Autodesk Inventor part; units mm, degrees
ref_plane "dia1_XY" through (-3.175, 3.9624, 0) normal (1, 0, 0) x (0, 0, -1)
ref_plane "dia1_YZ" through (-3.175, 3.9624, 0) normal (0, 0, -1) x (0, 1, 0)
ref_plane "dia1_ZX" through (-3.175, 3.9624, 0) normal (0, 1, 0) x (1, 0, 0)
sketch "Sketch_1" plane through (0, 0, 0) normal (0, 0, 1) x (1, 0, 0)
  line L0 (114.1984, 0) -> (-3.175, 0)
  line L1 (-3.175, 0) -> (-3.175, 3.9624)
  line L2 (-3.175, 3.9624) -> (92.075, 3.9624)
  line L3 (92.075, 3.9624) -> (92.075, 13.5572)
  line L4 (92.075, 13.5572) -> (114.1984, 13.5572)
  line L5 (114.1984, 13.5572) -> (114.1984, 0)
  line L6 (114.1984, 0) -> (-3.175, 0)
revolve "Revolution1" add sketch "Sketch_1" angle 360 about axis through (114.1984, 0, 0) along (1, 0, 0)
sketch "Sketch_3" plane through (0, 0, 0) normal (0, 0, 1) x (1, 0, 0)
  line L0 (-3.175, 0) -> (-15.875, 0)
  line L1 (-15.875, 0) -> (-15.875, 3.3388)
  line L2 (-15.875, 3.3388) -> (-15.2451, 3.9688)
  line L3 (-15.2451, 3.9688) -> (-3.175, 3.9688)
  line L4 (-3.175, 3.9688) -> (-3.175, 0)
  line L5 (-3.175, 0) -> (-15.875, 0)
revolve "Revolution2" add sketch "Sketch_3" angle 360 about axis through (-3.175, 0, 0) along (1, 0, 0)
thread "Thread1"
sketch "Sketch_10" plane through (-3.175, 0, 0) normal (1, 0, 0) x (0, 0, -1)
  line L0 (-7.9248, -7.9248) -> (7.9248, -7.9248)
  line L1 (7.9248, -7.9248) -> (7.9248, 7.9248)
  line L2 (7.9248, 7.9248) -> (-7.9248, 7.9248)
  line L3 (-7.9248, 7.9248) -> (-7.9248, -7.9248)
  line L4 (-3.175, -3.9624) -> (3.175, -3.9624)
  line L5 (3.175, -3.9624) -> (3.175, 3.9624)
  line L6 (3.175, 3.9624) -> (-3.175, 3.9624)
  line L7 (-3.175, 3.9624) -> (-3.175, -3.9624)
extrude "Extrusion1" cut sketch "Sketch_10" along normal blind 3.175
ref_plane "dia1_XY" through (-3.175, 3.9624, 0) normal (1, 0, 0) x (0, 0, -1)
ref_plane "dia1_YZ" through (-3.175, 3.9624, 0) normal (0, 0, -1) x (0, 1, 0)
ref_plane "dia1_ZX" through (-3.175, 3.9624, 0) normal (0, 1, 0) x (1, 0, 0)
ref_plane "dia12_XY" through (0, 0, 14.1351) normal (1, 0, 0) x (0, 0, -1)
ref_plane "dia12_YZ" through (0, 0, 14.1351) normal (0, 0, -1) x (0, 1, 0)
ref_plane "dia12_ZX" through (0, 0, 14.1351) normal (0, 1, 0) x (1, 0, 0)
ref_plane "dia2_XY" through (-3.175, -3.9624, 0) normal (1, 0, 0) x (0, 0, -1)
ref_plane "dia2_YZ" through (-3.175, -3.9624, 0) normal (0, 0, -1) x (0, 1, 0)
ref_plane "dia2_ZX" through (-3.175, -3.9624, 0) normal (0, 1, 0) x (1, 0, 0)
ref_plane "dia22_XY" through (0, 0, -14.1351) normal (1, 0, 0) x (0, 0, -1)
ref_plane "dia22_YZ" through (0, 0, -14.1351) normal (0, 0, -1) x (0, 1, 0)
ref_plane "dia22_ZX" through (0, 0, -14.1351) normal (0, 1, 0) x (1, 0, 0)
ref_plane "rl1_XY" through (-15.875, 0, 0) normal (1, 0, 0) x (0, 0, -1)
ref_plane "rl1_YZ" through (-15.875, 0, 0) normal (0, 0, -1) x (0, 1, 0)
ref_plane "rl1_ZX" through (-15.875, 0, 0) normal (0, 1, 0) x (1, 0, 0)
ref_plane "rl2_XY" through (-3.175, 0, 0) normal (1, 0, 0) x (0, 0, -1)
ref_plane "rl2_YZ" through (-3.175, 0, 0) normal (0, 0, -1) x (0, 1, 0)
ref_plane "rl2_ZX" through (-3.175, 0, 0) normal (0, 1, 0) x (1, 0, 0)
ref_plane "rod_cp_XY" through (0, 0, 0) normal (1, 0, 0) x (0, 0, -1)
ref_plane "rod_cp_YZ" through (0, 0, 0) normal (0, 0, -1) x (0, 1, 0)
ref_plane "rod_cp_ZX" through (0, 0, 0) normal (0, 1, 0) x (1, 0, 0)
ref_plane "thd1_XY" through (-15.875, 3.9688, 0) normal (1, 0, 0) x (0, 0, -1)
ref_plane "thd1_YZ" through (-15.875, 3.9688, 0) normal (0, 0, -1) x (0, 1, 0)
ref_plane "thd1_ZX" through (-15.875, 3.9688, 0) normal (0, 1, 0) x (1, 0, 0)
ref_plane "thd2_XY" through (-15.875, -3.9688, 0) normal (1, 0, 0) x (0, 0, -1)
ref_plane "thd2_YZ" through (-15.875, -3.9688, 0) normal (0, 0, -1) x (0, 1, 0)
ref_plane "thd2_ZX" through (-15.875, -3.9688, 0) normal (0, 1, 0) x (1, 0, 0)
ref_plane "to_rod_clevis_XY" through (-20.701, 0, 0) normal (1, 0, 0) x (0, 0, -1)
ref_plane "to_rod_clevis_YZ" through (-20.701, 0, 0) normal (0, 0, -1) x (0, 1, 0)
ref_plane "to_rod_clevis_ZX" through (-20.701, 0, 0) normal (0, 1, 0) x (1, 0, 0)
ref_plane "wf1_XY" through (-3.175, 0, 0) normal (1, 0, 0) x (0, 0, -1)
ref_plane "wf1_YZ" through (-3.175, 0, 0) normal (0, 0, -1) x (0, 1, 0)
ref_plane "wf1_ZX" through (-3.175, 0, 0) normal (0, 1, 0) x (1, 0, 0)
ref_plane "wf2_XY" through (0, 0, 0) normal (1, 0, 0) x (0, 0, -1)
ref_plane "wf2_YZ" through (0, 0, 0) normal (0, 0, -1) x (0, 1, 0)
ref_plane "wf2_ZX" through (0, 0, 0) normal (0, 1, 0) x (1, 0, 0)
ref_plane "wfw1_XY" through (-3.175, 0, -3.175) normal (0, 1, 0) x (1, 0, 0)
ref_plane "wfw1_YZ" through (-3.175, 0, -3.175) normal (1, 0, 0) x (0, 0, -1)
ref_plane "wfw1_ZX" through (-3.175, 0, -3.175) normal (0, 0, -1) x (0, 1, 0)
ref_plane "wfw2_XY" through (-3.175, 0, 3.175) normal (0, 1, 0) x (1, 0, 0)
ref_plane "wfw2_YZ" through (-3.175, 0, 3.175) normal (1, 0, 0) x (0, 0, -1)
ref_plane "wfw2_ZX" through (-3.175, 0, 3.175) normal (0, 0, -1) x (0, 1, 0)
properties part number "SR-092-DPY0000_rod"
The model under review builds one solid part; all positions refer to its coordinate system, in mm. A direction names the side the tool comes from. Round coordinates to 2 decimals unless told otherwise and drop trailing zeros. Loops run counter-clockwise (first coordinate to the right, second up) from the corner with the lowest first, then second, coordinate; pieces in that order, holes last. Notation, with made-up numbers: (23, -32.5) -> (58, -32.5) arc R17 cw to (58, -23.5) -> close; hole circle Ø11 at (15.25, -20). An arc over 180 degrees is marked (long way). Answer as a JSON object with one key per item and string values. Group by question number.
1) We need section A-A on z = 0. Write out the cut boundary in (x, y) (3 decimals), then the cut area to 3 significant figures.
2) Mouldability with a two-part tool opening along X and no side actions: class faces 4 (the face through (-9.126, 3.666, -1.52)), 5 (the face through (92.075, 3, -3)), 6 (the face through (-2, 0, -3.175)) as released by +X, released by -X, zero draft, split by the parting line, or undercut.
3) We need section B-B on y = 0. Write out the cut boundary in (x, z) (3 decimals), then the cut area to 3 significant figures.
4) For line 1 (X direction, y = -9, z = 4.5) (3 decimals); line 2 (Z direction, x = -7, y = 0.5); line 3 (Y direction, x = 47.5, z = -0.25), list the stretches that pass through material, from the lowest coordinate up. Write a range as [from, to].
5) We need section C-C on x = 84. Write out the cut boundary in (y, z), then the cut area to 3 significant figures.
6) For pin 1 Ø1.6 at (x, y) = (-2, -1) entering from -Z (3 decimals); pin 2 Ø2 at (x, y) = (17.5, -4.5) entering from -Z; pin 3 Ø5 at (y, z) = (-9.5, 0.5) entering from -X (3 decimals), all flat-tipped, find the tip position at first contact; note any pin that passes through.
7) For faces 1 (the face through (-2, 0, 3.175)), 2 (the face through (114.198, 0, 0)), 3 (the face through (45.12, -0.52, 3.93)), list the 3-axis set-ups (+Z, -Z, +X, -X, +Y, -Y) from which the entire face can be reached by the end or side of a thin tool; tool diameter is ignored.
8) We need section D-D on y = -9. Write out the cut boundary in (x, z) (3 decimals), then the cut area to 3 significant figures.
Result set:
{
 "1": {"outline": "(-15.875, -3.339) -> (-15.245, -3.969) -> (-3.175, -3.969) -> (-3.175, -3.962) -> (92.075, -3.962) -> (92.075, -13.557) -> (114.198, -13.557) -> (114.198, 13.557) -> (92.075, 13.557) -> (92.075, 3.962) -> (-3.175, 3.962) -> (-3.175, 3.969) -> (-15.245, 3.969) -> (-15.875, 3.339) -> close", "area": "1,460 mm²"},
 "2": {"face 4": "zero draft", "face 5": "released by -X", "face 6": "undercut"},
 "3": {"outline": "(-15.875, -3.339) -> (-15.245, -3.969) -> (-3.175, -3.969) -> (-3.175, -3.175) -> (0, -3.175) -> (0, -3.962) -> (92.075, -3.962) -> (92.075, -13.557) -> (114.198, -13.557) -> (114.198, 13.557) -> (92.075, 13.557) -> (92.075, 3.962) -> (0, 3.962) -> (0, 3.175) -> (-3.175, 3.175) -> (-3.175, 3.969) -> (-15.245, 3.969) -> (-15.875, 3.339) -> close", "area": "1,450 mm²"},
 "4": {"line 1": "[92.075, 114.198]", "line 2": "[-3.94, 3.94]", "line 3": "[-3.95, 3.95]"},
 "5": {"outline": "circle Ø7.92 at (0, 0)", "area": "49.3 mm²"},
 "6": {"pin 1": "z = -3.175", "pin 2": "z = -1.86", "pin 3": "x = 92.075"},
 "7": {"face 1": "+Z, +Y, -Y", "face 2": "+Z, -Z, +X, +Y, -Y", "face 3": "-X"},
 "8": {"outline": "(92.075, -10.139) -> (114.198, -10.139) -> (114.198, 10.139) -> (92.075, 10.139) -> close", "area": "449 mm²"}
}
